Source: CAD feature listing. Evaluate the final solid. Frame: model axes, mm. Face numbers are marked on the shaded views. A direction names the side the tool comes from. Coordinates: 2 decimals unless noted, no trailing zeros. Write each loop counter-clockwise with the first axis right and the second up, starting at its lowest first coordinate (ties: lowest second). Pieces come first, ordered by that corner, then holes. Notation, with made-up numbers: M 18,44 L 40,44 A27 cw 40,64 Z; hole C -35.5,-18.5 d4. An arc over 180 degrees is marked long. Answer as CSV lines item,"result". Start each with the question number.
1. Section B-B on x = -11. Return the cut outline in (y, z).
2. Section A-A on x = 68.5. Return the cut outline in (y, z).
3. Contact query for flat-ended pins moving along their axis: pin 1 Ø1.4 at (x, y) = (-13, 0.5) entering from +Z; pin 2 Ø3 at (y, z) = (-19.5, 12.5) entering from -X; pin 3 Ø8 at (x, z) = (5, -11) entering from -Y. Output: stop coordinate, or through.
4. Section C-C on x = 6. Return the cut outline in (y, z), plus the area to 3 significant figures.
5. Reachability of the marked faces 1, 2 and 3 from +Z, -Z, +X, -X, +Y, -Y: full face, straight path, thin tool, end or side. Return the list, or none.
6. Line query: probe 1 along Z at (x, y) = (68.5, -27.8); probe 2 along Y at (x, z) = (-13.5, -3.5); probe 3 along X at (y, z) = (-18.5, 6). Output: solid intervals per line, ascending. Write a range as [from, to].
```python
from build123d import *

# Parameters (mm, degrees)
F1_DEPTH = 16
F3_DEPTH = 12.5
F5_DEPTH = 12.5
F6_W     = 13
F6_H     = 7.5
F7_DEPTH = 12.5
F8_R     = 3.5
F9_DEPTH = 12.5
F10_R    = 0.2


with BuildPart() as f1:
    # F0 (on Top) → F1 (new body, symmetric)
    with BuildSketch(Plane.XY):
        with BuildLine():
            Line((-27.5, -1), (27.5, -1))
            ThreePointArc((27.5, -1), (48.3865985742, -9.0362658643), (58.5, -29))
            Line((58.5, -29), (76.5, -29))
            Line((76.5, -29), (76.5, -27))
            Line((76.5, -27), (60.2566787083, -27))
            ThreePointArc((60.2566787083, -27), (49.0464614264, -6.9539102055), (27.5, 1))
            Line((27.5, 1), (-27.5, 1))
            Line((-27.5, 1), (-27.5, -1))
        make_face()
    extrude(amount=F1_DEPTH, both=True)

    # F2 (on face) → F3 (cut, symmetric)
    with BuildSketch(Plane.XZ.offset(29)):
        with BuildLine():
            Line((76.5, 0), (76.5, 16))
            Line((76.5, 16), (73.5, 16))
            ThreePointArc((73.5, 16), (75.7435215896, 8.139410298), (76.5, 0))
        make_face()
        with BuildLine():
            Line((76.5, -16), (76.5, 0))
            ThreePointArc((76.5, 0), (75.7435215896, -8.139410298), (73.5, -16))
            Line((73.5, -16), (76.5, -16))
        make_face()
    extrude(amount=F3_DEPTH, both=True, mode=Mode.SUBTRACT)

    # F4 (on face) → F5 (cut, symmetric)
    with BuildSketch(Plane(origin=(0, 1, 0), x_dir=(-1, 0, 0), z_dir=(0, 1, 0))):
        with BuildLine():
            Line((27.5, -16), (27.5, -3.42e-08))
            ThreePointArc((27.5, -3.42e-08), (26.2208873777, -8.3815273234), (22.5, -16))
            Line((22.5, -16), (27.5, -16))
        make_face()
        with BuildLine():
            Line((27.5, -3.42e-08), (27.5, 16))
            Line((27.5, 16), (22.5, 16))
            ThreePointArc((22.5, 16), (26.2208873879, 8.3815272908), (27.5, -3.42e-08))
        make_face()
    extrude(amount=F5_DEPTH, both=True, mode=Mode.SUBTRACT)

    # F6 (on face) → F7 (cut, symmetric)
    with BuildSketch(Plane(origin=(0, 1, 0), x_dir=(-1, 0, 0), z_dir=(0, 1, 0))):
        with Locations((10, -12.25)):
            Rectangle(F6_W, F6_H)
        with Locations((10, 12.25)):
            Rectangle(F6_W, F6_H)
    extrude(amount=F7_DEPTH, both=True, mode=Mode.SUBTRACT)

    # F8 (on face) → F9 (cut, symmetric)
    with BuildSketch(Plane(origin=(0, -27, 0), x_dir=(-1, 0, 0), z_dir=(0, 1, 0))):
        with Locations((-68.5, 0)):
            Circle(F8_R)
    extrude(amount=F9_DEPTH, both=True, mode=Mode.SUBTRACT)

    # F10
    f10_edges = [f1.edges().sort_by_distance(p)[0] for p in [
        (76.5, -27, 0),
        (66.878339, -27, 16),
        (66.878339, -27, -16),
        (60.256679, -27, 0),
        (72, -27, 0),
        (49.046461, -6.95391, -16),
        (27.5, 1, 0),
        (49.046461, -6.95391, 16),
        (12, 1, 16),
        (-3.5, 1, 12.25),
        (-10, 1, 8.5),
        (-16.5, 1, 12.25),
        (-19.5, 1, 16),
        (-27.5, 1, 0),
        (-19.5, 1, -16),
        (-16.5, 1, -12.25),
        (-10, 1, -8.5),
        (-3.5, 1, -12.25),
        (12, 1, -16),
    ]]
    fillet(f10_edges, radius=F10_R)


solid = f1.part
```
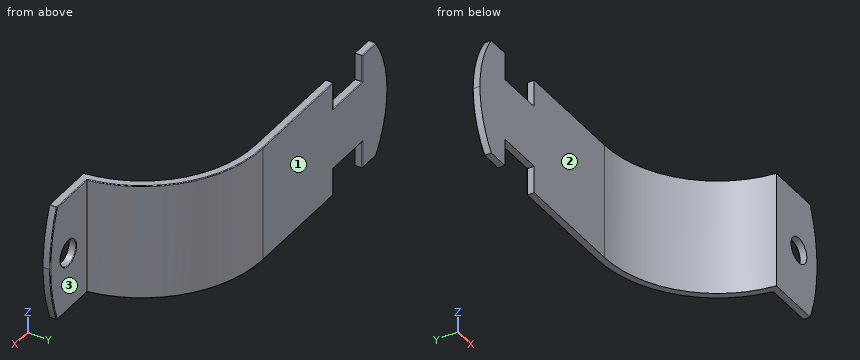
Values:
1,outline,"M -1,-8.5 L 0.8,-8.5 A0.2 ccw 1,-8.3 L 1,8.3 A0.2 ccw 0.8,8.5 L -1,8.5 Z"
2,outline,"M -29,-16 L -27.2,-16 A0.2 ccw -27,-15.8 L -27,-3.7 A0.2 ccw -27.2,-3.5 L -29,-3.5 Z; M -29,3.5 L -27.2,3.5 A0.2 ccw -27,3.7 L -27,15.8 A0.2 ccw -27.2,16 L -29,16 Z"
3,pin 1,"z = 8.5"
3,pin 2,"x = 55.26"
3,pin 3,"y = -1"
4,outline,"M -1,-16 L 0.8,-16 A0.2 ccw 1,-15.8 L 1,15.8 A0.2 ccw 0.8,16 L -1,16 Z"
4,area,"64.0 mm²"
5,face 1,"+Z, -Z, +X, -X, +Y"
5,face 2,"+Z, -Z, -X, -Y"
5,face 3,"+Z, -Z, +X, +Y"
6,probe 1,"[-16, -3.5], [3.5, 16]"
6,probe 2,"[-1, 1]"
6,probe 3,"[55.51, 57.72]"
